Source: CAD feature listing. Evaluate the final solid. Frame: model axes, mm. Face numbers are marked on the shaded views. A direction names the side the tool comes from. Round coordinates to 2 decimals unless told otherwise and drop trailing zeros. Write each loop counter-clockwise with the first axis right and the second up, starting at its lowest first coordinate (ties: lowest second). Pieces come first, ordered by that corner, then holes.
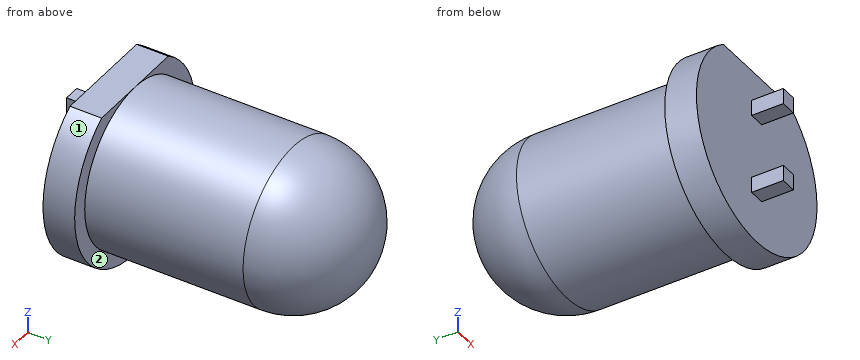
Autodesk Inventor part; units mm, degrees
ref_plane "YZ Plane" through (0, 0, 0) normal (1, 0, 0) x (0, 1, 0)
ref_plane "XZ Plane" through (0, 0, 0) normal (0, 1, 0) x (-1, 0, 0)
ref_plane "XY Plane" through (0, 0, 0) normal (0, 0, 1) x (1, 0, 0)
sketch "Sketch1" plane through (0, 0, 0) normal (0, 1, 0) x (-1, 0, 0)
  arc A0 (-1.6583, 2.5) -> (1.6583, 2.5) centre (0, 0) ccw
  circle A1 centre (0, 0) radius 2.5
  line L0 (-1.6583, 2.5) -> (1.6583, 2.5)
  dimension "d0" = 6
  dimension "d1" = 5
extrude "Extrusion3" add sketch "Sketch1" along normal blind 1 contours A1 | L0 A0
sketch "Sketch2" plane through (0, 1, 0) normal (0, 1, 0) x (1, 0, 0)
  circle A0 centre (0, 0) radius 2.5
  point P0 (0, -2.5)
extrude "Extrusion5" add sketch "Sketch2" along normal blind 7.5
fillet "Fillet2" radius 2.5 1 edges at (-2.5, 8.5, 0)
sketch "Sketch3" plane through (0, 0, 0) normal (0, -1, 0) x (1, 0, 0)
  line L0 (-0.25, 1.52) -> (0.25, 1.52)
  line L1 (0.25, 1.52) -> (0.25, 1.02)
  line L2 (0.25, 1.02) -> (-0.25, 1.02)
  line L3 (-0.25, 1.02) -> (-0.25, 1.52)
  line L4 (-0.25, -1.02) -> (0.25, -1.02)
  line L5 (0.25, -1.02) -> (0.25, -1.52)
  line L6 (0.25, -1.52) -> (-0.25, -1.52)
  line L7 (-0.25, -1.52) -> (-0.25, -1.02)
  line L8 (-0.3964, 1.27) -> (0.6648, 1.27) construction
  line L9 (-0.5129, -1.27) -> (0.7016, -1.27) construction
  line L10 (-1.0602, 0) -> (0.7998, 0) construction
  point P0 (0, 0)
  point P1 (0.25, -1.27)
  point P2 (0.25, 1.27)
  point P3 (0, 1.02)
  dimension "d18" = 0.5
  dimension "d19" = 2.54
extrude "Extrusion6" add sketch "Sketch3" along normal blind 1
properties part number "LED"
Q1. Set-up query: the marked faces 1 and 2. Return all of +Z, -Z, +X, -X, +Y, -Y with unobstructed straight access to the full face (end or side cutting, diameter ignored); none if empty.
Q2. Section query A-A, the plane z = 0. Output: boundary loops of the cut face in (x, y).
Q3. Section query C-C, the plane y = 3. Output: boundary loops of the cut face in (x, z).
Q4. Line query: line 1 (Z direction, x = 1.1, y = 8); line 2 (Y direction, x = 0.1, z = -2.65); line 3 (X direction, y = 2.25, z = -0.05). Output: solid intervals per line, ascending.
Q5. Pin query (flat end, axial travel): P1, Ø1, axis at x = -0.5, y = 3, coming from the +Z side; P2, Ø3, axis at x = 0, y = 4.5, coming from the -Z side. Return the tip coordinate at first contact, or that it passes through.
Q6. Section query B-B, the plane x = -1.8. Output: boundary loops of the cut face in (y, z), and give its area (3 significant figures).
Q7. Section query D-D, the plane y = 0.5. Output: boundary loops of the cut face in (x, z).
Filled in:
1. face 1: +Y, -Y
1. face 2: +Y
2. outline: (-3, 0) - (3, 0) - (3, 1) - (2.5, 1) - (2.5, 6) arc R2.5 ccw to (-2.5, 6) - (-2.5, 1) - (-3, 1) - close
3. outline: circle Ø5 at (0, 0)
4. line 1: z = -1.02 to 1.02
4. line 2: y = 0 to 1
4. line 3: x = -2.5 to 2.5
5. P1: stops at z = 2.5
5. P2: stops at z = -2.5
6. outline: (0, -2.4) - (1, -2.4) - (1, -1.73) - (6, -1.73) arc R1.73 ccw to (6, 1.73) - (1, 1.73) - (1, 2.4) - (0, 2.4) - close
6. area: 26.9 mm2
7. outline: (-1.66, 2.5) arc R3 ccw (long way) to (1.66, 2.5) - close
